Input: part model. Units: mm. Frame: model coordinates. A direction names the side the tool comes from. Give positions to 0.01 mm unless a question says otherwise; leave off trailing zeros. Order: outer loops, then holes, each group sorted by start corner. A loop starts at its lowest first (then second) coordinate and runs counter-clockwise, first axis right, second up. Notation, with made-up numbers: (43.25, 89) - (83.25, 89) arc R17 ccw to (83.25, 122) - close; hole circle Ø1 at (2, -32). An arc over 180 degrees is marked (long way). Answer in a Markdown table with one row per item. Add a question column.
1. Section query A-A on x = 0. Return loops of the section in (y, z).
2. Section query C-C on y = 1.25. Return loops of the section in (x, z), and give its area (3 significant figures).
3. Access query for faces 5 (the face through (-16.751, 7.181, -0.602)), 6 (the face through (-3, 9.608, 12)), 7 (the face through (-10.3, 7, -8.4)). Directions: +Z, -Z, +X, -X, +Y, -Y. A direction counts if a zero-diameter tool reaches every point of the face in a straight line with its end or side. Return the directions, or none.
4. Ray query, line 1 (X direction, y = 8, z = 0); line 2 (X direction, y = 3.75, z = 0); line 3 (X direction, y = 6.5, z = 0). Return the intervals inside material, ascending. Write a range as [from, to].
5. Section query D-D on y = 8.75. Count the separate pieces of the cut face and the enclosed holes in it, and give its area (3 significant figures).
6. Section query B-B on z = 3. Return loops of the section in (x, y).
7. Mould query, pull axis Z, two halves, no side actions, for faces 1 (the face through (14.428, 6.634, 8.755)), 2 (the face through (-3.776, 9.539, 13.508)), 3 (the face through (13.198, 7.181, 10.334)), 4 (the face through (10.916, 8.688, -8.692)). Classes: released by +Z, released by -Z, zero draft, split by the parting line, or undercut.
8. Contact query for flat-ended pins moving along their axis: pin 1 (0.7 mm diameter, centred on x = -5, z = -11.5, fed in from +Y); pin 2 (2 mm diameter, centred on y = 8.5, z = -2, fed in from +X); pin 3 (2 mm diameter, centred on x = -10.5, z = -9, fed in from -Y); pin 4 (4 mm diameter, centred on x = 10.5, z = -8.5, fed in from -Y). Output: stop coordinate, or through.
```python
from build123d import *

# Parameters (mm, degrees)
ESQUISSE1_R                      = 12.05
ESQUISSE1_R_2                    = 10.05
BASE_DEPTH                       = 10
BOSS_TIGE_DEPTH                  = 2
CONGE_TIGE_R                     = 0.2
REP_SUPPORT_TIGE_COUNT           = 5
CONGE_TIGE_OF_REP_SUPPORT_TIGE_R = 0.2
BOSS_EXTRU_1_DEPTH               = 3
CONG_1_R                         = 0.5


with BuildPart() as part:
    # Esquisse1 → BASE (new body)
    with BuildSketch(Plane(origin=(0, 0, 0), x_dir=(1, 0, 0), z_dir=(0, 1, 0))):
        with Locations(Location((0, 0, 0), (0, 0, 270))):
            Circle(ESQUISSE1_R)
        with Locations(Location((0, 0, 0), (0, 0, 270))):
            Circle(ESQUISSE1_R_2, mode=Mode.SUBTRACT)
    extrude(amount=BASE_DEPTH)

    # Esquisse7 → BOSS TIGE (add)
    with BuildSketch(Plane(origin=(-2.523980967, 0, 0.624115435), x_dir=(-0.2400443980205285, -8.560907231219602e-15, -0.9707619105522024), z_dir=(0.9707619105522023, 0, -0.24004439802052846))):
        with BuildLine():
            Line((14.022631891, 9.608391049), (11.415742159, 9.608391049))
            Line((11.415742159, 9.608391049), (11.415742159, 4.685414017))
            Line((11.415742159, 4.685414017), (18.629521623, 4.685414017))
            Line((18.629521623, 4.685414017), (18.629521623, 9.608391049))
            Line((18.629521623, 9.608391049), (16.022631891, 9.608391049))
            Line((16.022631891, 9.608391049), (16.302913172, 8.020618644))
            ThreePointArc((16.302913172, 8.020618644), (15.022631891, 5.596902533), (13.742350611, 8.020618644))
            Line((13.742350611, 8.020618644), (14.022631891, 9.608391049))
        make_face()
    boss_tige = extrude(amount=BOSS_TIGE_DEPTH)

    # CONGE TIGE
    conge_tige_edges = [part.edges().sort_by_distance(p)[0] for p in [
        (-4.919273288, 9.608391049, -13.228565889),
        (-5.399362084, 9.608391049, -15.17008971),
    ]]
    fillet(conge_tige_edges, radius=CONGE_TIGE_R)

    # REP SUPPORT TIGE: BOSS TIGE ×5 about axis
    rep_support_tige_axis = Axis((0, 0, 0), (0, 1, 0))
    for i in range(1, REP_SUPPORT_TIGE_COUNT):
        add(boss_tige.rotate(rep_support_tige_axis, i * 360 / REP_SUPPORT_TIGE_COUNT))

    # CONGE TIGE of REP SUPPORT TIGE
    conge_tige_of_rep_support_tige_edges = [part.edges().sort_by_distance(p)[0] for p in [
        (-14.101252836, 9.608391049, 0.590655245),
        (-16.096107314, 9.608391049, 0.447282967),
        (-3.795780249, 9.608391049, 13.593610906),
        (-4.548579323, 9.608391049, 15.446525786),
        (11.755331628, 9.608391049, 7.810658325),
        (13.284930692, 9.608391049, 9.099194977),
        (11.060974744, 9.608391049, -8.766358587),
        (12.759118029, 9.608391049, -9.82291402),
    ]]
    fillet(conge_tige_of_rep_support_tige_edges, radius=CONGE_TIGE_OF_REP_SUPPORT_TIGE_R)

    # Esquisse8 → Boss.-Extru.1 (add)
    with BuildSketch(Plane(origin=(0, 10, 0), x_dir=(1, 0, 0), z_dir=(0, 1, 0))):
        with BuildLine():
            Line((-8.268421395, 8.757415667), (-7.703456323, 8.300627196))
            ThreePointArc((-7.703456323, 8.300627196), (-8.759173713, 7.17778009), (-9.652653966, 5.92198637))
            Line((-9.652653966, 5.92198637), (-10.190441919, 6.359674812))
            Line((-10.190441919, 6.359674812), (-9.690340196, 6.974149988))
            Line((-9.690340196, 6.974149988), (-10.694246531, 7.791197297))
            Line((-10.694246531, 7.791197297), (-11.194348255, 7.176722121))
            Line((-11.194348255, 7.176722121), (-11.732136208, 7.614410563))
            Line((-11.732136208, 7.614410563), (-9.79837654, 9.990421794))
            Line((-9.79837654, 9.990421794), (-9.28435206, 9.559462499))
            Line((-9.28435206, 9.559462499), (-9.775272229, 8.937627422))
            Line((-9.775272229, 8.937627422), (-8.759341564, 8.13558059))
            Line((-8.759341564, 8.13558059), (-8.268421395, 8.757415667))
        make_face()
    extrude(amount=-BOSS_EXTRU_1_DEPTH)

    # Cong_1
    cong_1_edges = [part.edges().sort_by_distance(p)[0] for p in [
        (-9.304844667, 7, -8.566238952),
        (-10.235385675, 7, -7.417745099),
        (-9.304844667, 10, -8.566238952),
        (-10.235385675, 10, -7.417745099),
    ]]
    fillet(cong_1_edges, radius=CONG_1_R)


solid = part.part
```
Answer:
| question | item | result |
|---|---|---|
| 1 | outline | (0, -12.05) - (10, -12.05) - (10, -10.05) - (0, -10.05) - close; (0, 10.05) - (10, 10.05) - (10, 12.05) - (0, 12.05) - close |
| 2 | outline | circle Ø24.1 at (0, 0); hole circle Ø20.1 at (0, 0) |
| 2 | area | 139 mm² |
| 3 | face 5 | -Z, +Y, -Y |
| 3 | face 6 | +Z, -X, +Y |
| 3 | face 7 | -Z, -X, -Y |
| 4 | line 1 | x = [-18.68, -16.36], [-13.76, -10.05], [10.05, 12.05] |
| 4 | line 2 | x = [-12.05, -10.05], [10.05, 12.05] |
| 4 | line 3 | x = [-18.68, -16.47], [-13.65, -10.05], [10.05, 12.05] |
| 5 | separate pieces | 6 |
| 5 | enclosed holes | 1 |
| 5 | area | 187 mm² |
| 6 | outline | (-11.67, 0) - (-9.59, 0) - (-9.59, 10) - (-11.67, 10) - close; (9.59, 0) - (11.67, 0) - (11.67, 10) - (9.59, 10) - close |
| 7 | face 1 | undercut |
| 7 | face 2 | undercut |
| 7 | face 3 | released by +Z |
| 7 | face 4 | released by -Z |
| 8 | pin 1 | stops at y = 9.61 |
| 8 | pin 2 | stops at x = 12.01 |
| 8 | pin 3 | stops at y = 7 |
| 8 | pin 4 | stops at y = 0 |
